Geometry: see drawing. Coordinates: mm, zero at the bounding-box minimum. A direction names the side the tool comes from. Coordinates: 2 decimals unless noted, no trailing zeros. Loops run counter-clockwise (first coordinate to the right, second up) from the corner with the lowest first, then second, coordinate; pieces in that order, holes last. Notation, with made-up numbers: (-17, 68.25) - (9, 68.25) arc R14 ccw to (9, 83.25) - close; hole circle Ø7 at (39, 8.25). An arc over 180 degrees is marked (long way). Use one line per item in the form item = value.
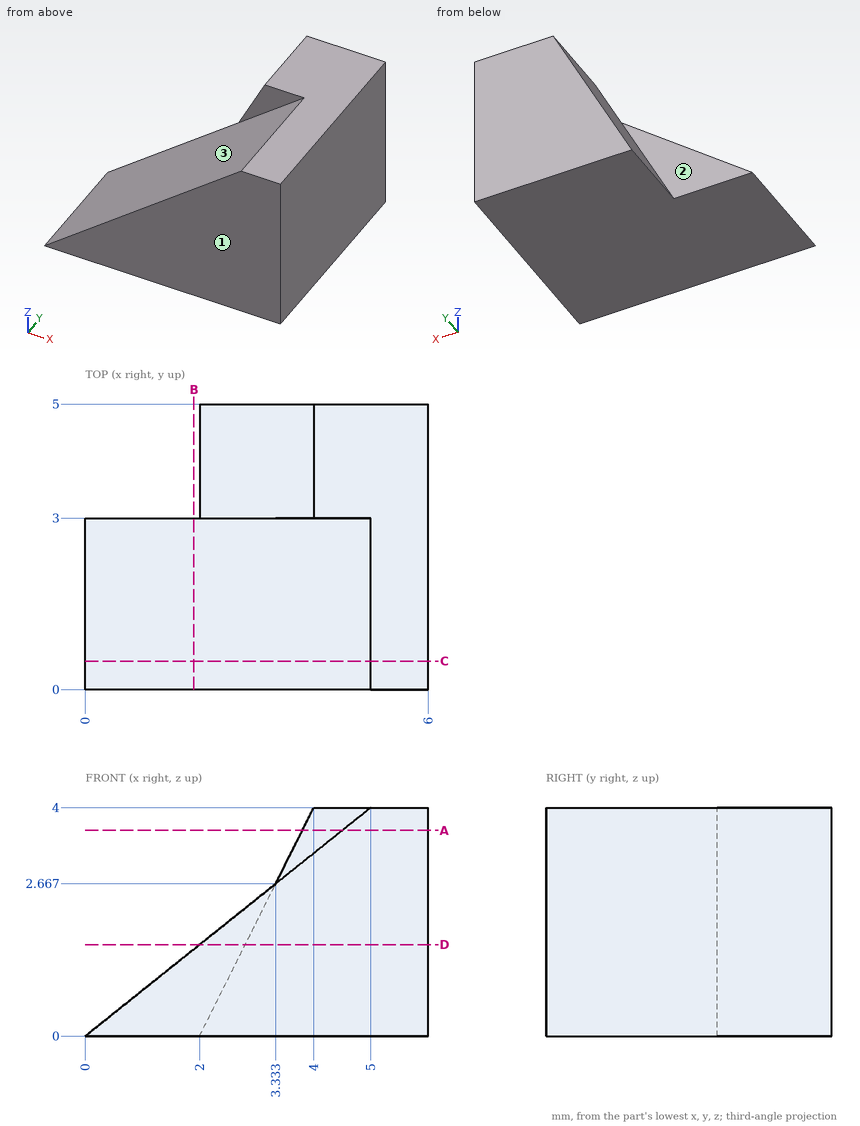
Q1. Cut plane C-C, the plane y = 0.5. Return loops of the section in (x, z), then the cut area to 3 significant figures.
Check values:
outline = (0, 0) - (6, 0) - (6, 4) - (5, 4) - close
area = 14.0 mm²
Q2. Cut plane B-B, the plane x = 1.9. Return loops of the section in (y, z).
Check values:
outline = (0, 0) - (3, 0) - (3, 1.52) - (0, 1.52) - close
Q3. Cut plane D-D, the plane z = 1.6. Return loops of the section in (x, y).
Check values:
outline = (2, 0) - (6, 0) - (6, 5) - (2.8, 5) - (2.8, 3) - (2, 3) - close
Q4. Ray query, line 1 along Y through (x, z) = (2.05, 0.2); line 2 along X through (y, z) = (4, 2); line 3 along X through (y, z) = (0.95, 0.6). Return the intervals inside material, ascending. Write a range as [from, to].
Check values:
line_1 = [0, 3]
line_2 = [3, 6]
line_3 = [0.75, 6]
Q5. Cut plane A-A, the plane z = 3.6. Return loops of the section in (x, y).
Check values:
outline = (3.8, 3) - (4.5, 3) - (4.5, 0) - (6, 0) - (6, 5) - (3.8, 5) - close
Q6. First-contact query: P1, Ø3, axis at x = 5, y = 3, coming from the -Z side; P2, Ø1.5, axis at y = 1, z = 2, coming from the -X side; P3, Ø1.3, axis at x = 1, z = 0.5, coming from the +Y side. Flat tips, straight axial feed; report the tip coordinate or a pass-through.
Check values:
P1 = 0
P2 = 1.56
P3 = 3
Q7. Set-up query: the marked faces 1, 2 and 3. Return all of +Z, -Z, +X, -X, +Y, -Y with unobstructed straight access to the full face (end or side cutting, diameter ignored); none if empty.
Check values:
face_1 = +Z, -Z, +X, -X, -Y
face_2 = +Z, -X, +Y
face_3 = +Z, -X, -Y
